Verification items for this drawing (mm, ordinates from the low corner). Give positions to 0.01 mm unless a question says otherwise; leave off trailing zeros. Loops run counter-clockwise (first coordinate to the right, second up) from the corner with the lowest first, then second, coordinate; pieces in that order, holes last. Notation, with made-up numbers: (1.5, 52) -> (46.5, 52) arc R9 cw to (46.5, 66) -> close; hole circle Ø3 at (-37, 30). An arc over 180 degrees is marked (long way). Write item = value, one per line.
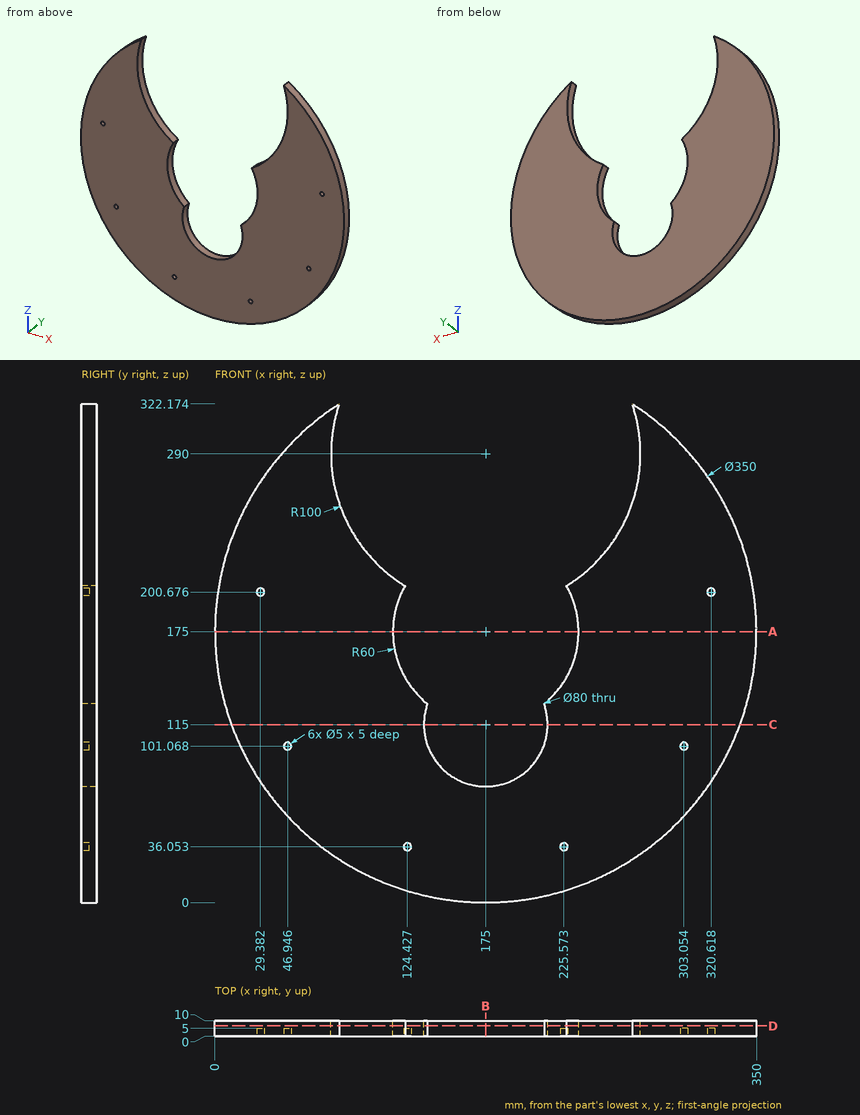
Item 1: Thickness scan on L1, parallel to X at y = 7.75, z = 255 (1 decimal); L2, parallel to X at y = 7.75, z = 138.5; L3, parallel to Z at x = 177.5, y = 1. Record the ranges inside material, lowest first. Write a range as [from, to].
Answer:
L1 = [19.4, 81.3], [268.7, 330.6]
L2 = [3.85, 127.38], [222.62, 346.15]
L3 = [0.02, 75.08]
Item 2: Gauge pin test, flat ends, axial feed: pin 1 (1.5 mm diameter, centred on x = 47, z = 100.5, fed in from -Y); pin 2 (1 mm diameter, centred on x = 260.5, y = 2.5, fed in from +Z); pin 3 (5 mm diameter, centred on y = 1.5, z = 273.5, fed in from +X). Record the tip position at first contact, or that the pin passes through.
Answer:
pin_1 = 5
pin_2 = 238.97
pin_3 = 321.32
Item 3: Section check D-D, the plane y = 6.5. Record the cut outline in (x, z), plus the area to 3 significant figures.
Answer:
outline = (80.32, 322.17) arc R175 ccw (long way) to (269.68, 322.17) arc R100 cw to (227.15, 204.67) arc R60 cw to (212.71, 128.33) arc R40 cw (long way) to (137.29, 128.33) arc R60 cw to (122.85, 204.67) arc R100 cw to start
area = 59,700 mm^2
Item 4: Section check B-B, the plane x = 175. Record the cut outline in (y, z), plus the area to 3 significant figures.
Answer:
outline = (0, 0) -> (10, 0) -> (10, 75) -> (0, 75) -> close
area = 750 mm^2
Item 5: Section check A-A, the plane z = 175. Record the cut outline in (x, y).
Answer:
outline = (0, 0) -> (115, 0) -> (115, 10) -> (0, 10) -> close; (235, 0) -> (350, 0) -> (350, 10) -> (235, 10) -> close
Item 6: Section check C-C, the plane z = 115. Record the cut outline in (x, y), plus the area to 3 significant figures.
Answer:
outline = (10.61, 0) -> (135, 0) -> (135, 10) -> (10.61, 10) -> close; (215, 0) -> (339.39, 0) -> (339.39, 10) -> (215, 10) -> close
area = 2,490 mm^2
